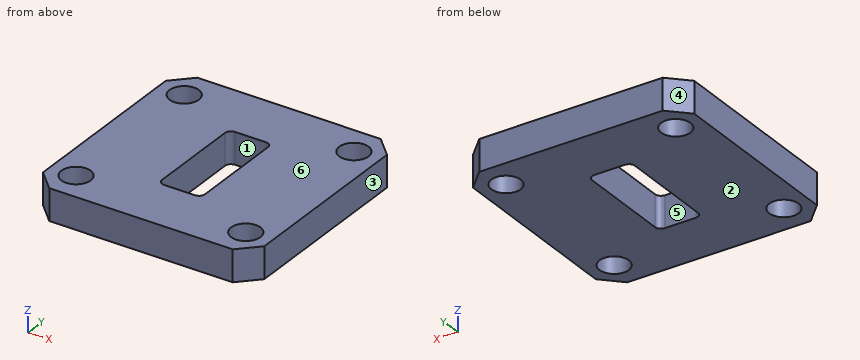
from build123d import *

# Parameters (mm, degrees)
F0_W     = 22.2504
F0_H     = 22.2504
F0_R     = 1.4732
F0_W_2   = 4.318
F0_H_2   = 10.668
F1_DEPTH = 3.175
F2_SIZE  = 1.905
F3_R     = 0.5969


with BuildPart() as f1:
    # F0 (on Top) → F1 (new body)
    with BuildSketch(Plane.XY):
        Rectangle(F0_W, F0_H)
        with Locations((-8.5344, -8.128)):
            Circle(F0_R, mode=Mode.SUBTRACT)
        with Locations((8.5344, -8.128)):
            Circle(F0_R, mode=Mode.SUBTRACT)
        with Locations((-8.5344, 8.128)):
            Circle(F0_R, mode=Mode.SUBTRACT)
        Rectangle(F0_W_2, F0_H_2, mode=Mode.SUBTRACT)
        with Locations((8.5344, 8.128)):
            Circle(F0_R, mode=Mode.SUBTRACT)
    extrude(amount=F1_DEPTH)

    # F2
    f2_edges = [f1.edges().sort_by_distance(p)[0] for p in [
        (-11.1252, -11.1252, 1.5875),
        (-11.1252, 11.1252, 1.5875),
        (11.1252, 11.1252, 1.5875),
        (11.1252, -11.1252, 1.5875),
    ]]
    chamfer(f2_edges, length=F2_SIZE)

    # F3
    f3_edges = [f1.edges().sort_by_distance(p)[0] for p in [
        (2.159, -5.334, 1.5875),
        (-2.159, -5.334, 1.5875),
        (-2.159, 5.334, 1.5875),
        (2.159, 5.334, 1.5875),
    ]]
    fillet(f3_edges, radius=F3_R)


solid = f1.part
Can you work these out from the model? Positions are in its coordinate system, mm. Face numbers are marked on the shaded views. A direction names the side the tool comes from. Round coordinates to 2 decimals unless told otherwise and drop trailing zeros. Loops run counter-clockwise (first coordinate to the right, second up) from the corner with the lowest first, then second, coordinate; pieces in that order, holes last. Notation, with made-up numbers: (50, -38) - (106, -38) arc R13 ccw to (106, -25) - close; hole circle Ø6 at (52.25, 7.25). An arc over 180 degrees is marked (long way). Write item = value, one per line. Start each with the question number.
(1) If we section it at B-B (y = -7.5): Please give me the cut outline in (x, z) (3 decimals), and give its area (3 significant figures).
(2) If I drill on probe 1 along X at (y, z) = (0.5, 1.6); probe 2 along Y at (x, z) = (-9, 2.65); probe 3 along X at (y, z) = (-9, 1.65), over which ranges is the centre line in solid material (lowest first)? Write a range as [from, to].
(3) If we section it at A-A (y = 0.5): Please give me the cut outline in (x, z) (3 decimals), and give its area (3 significant figures).
(4) If we section it at D-D (z = 0.75): Please give me the cut outline in (x, y).
(5) For the marked faces 5 and 6, which set-ups out of +Z, -Z, +X, -X, +Y, -Y let a thin tool reach every point of the face, with its end or its side?
(6) If we mould it in two halves opening along X, with no side actions, what happens to the marked faces 1, 2, 3 and 4? For each: released by +X, released by -X, zero draft, split by the parting line, or undercut.
(7) If we section it at C-C (x = 8): Please give me the cut outline in (y, z) (3 decimals).
(8) For P1, Ø1.8, axis at x = 8.53, y = 8.13, coming from the -Z side, with a flat end and sliding along its axis, tell me the tip position at first contact or that it passes through.
Ans:
q1.outline = (-11.125, 0) - (-9.867, 0) - (-9.867, 3.175) - (-11.125, 3.175) - close; (-7.202, 0) - (7.202, 0) - (7.202, 3.175) - (-7.202, 3.175) - close; (9.867, 0) - (11.125, 0) - (11.125, 3.175) - (9.867, 3.175) - close
q1.area = 53.7 mm²
q2.probe_1 = [-11.13, -2.16], [2.16, 11.13]
q2.probe_2 = [-11.13, -9.53], [-6.73, 6.73], [9.53, 11.13]
q2.probe_3 = [-11.13, -9.72], [-7.35, 7.35], [9.72, 11.13]
q3.outline = (-11.125, 0) - (-2.159, 0) - (-2.159, 3.175) - (-11.125, 3.175) - close; (2.159, 0) - (11.125, 0) - (11.125, 3.175) - (2.159, 3.175) - close
q3.area = 56.9 mm²
q4.outline = (-11.13, -9.22) - (-9.22, -11.13) - (9.22, -11.13) - (11.13, -9.22) - (11.13, 9.22) - (9.22, 11.13) - (-9.22, 11.13) - (-11.13, 9.22) - close; hole circle Ø2.95 at (-8.53, -8.13); hole circle Ø2.95 at (-8.53, 8.13); hole (-2.16, -4.74) arc R0.6 ccw to (-1.56, -5.33) - (1.56, -5.33) arc R0.6 ccw to (2.16, -4.74) - (2.16, 4.74) arc R0.6 ccw to (1.56, 5.33) - (-1.56, 5.33) arc R0.6 ccw to (-2.16, 4.74) - close; hole circle Ø2.95 at (8.53, -8.13); hole circle Ø2.95 at (8.53, 8.13)
q5.face_5 = +Z, -Z
q5.face_6 = +Z, +X, -X, +Y, -Y
q6.face_1 = undercut
q6.face_2 = zero draft
q6.face_3 = released by +X
q6.face_4 = released by -X
q7.outline = (-11.125, 0) - (-9.501, 0) - (-9.501, 3.175) - (-11.125, 3.175) - close; (-6.755, 0) - (6.755, 0) - (6.755, 3.175) - (-6.755, 3.175) - close; (9.501, 0) - (11.125, 0) - (11.125, 3.175) - (9.501, 3.175) - close
q8.P1 = through
